from build123d import *

# Parameters (mm, degrees)
F1_W     = 101.6
F1_H     = 101.6
F2_DEPTH = 50.8
F3_W     = 34.3186343089
F3_H     = 34.3186343089
F4_DEPTH = 46.228
F5_W     = 34.3186343089
F5_H     = 34.3186343089
F6_DEPTH = 45.974


# Not quite as in the source:
# - a variable given as a bare number and used for a length is read in inches; the dataset says mm whatever the document's units were


with BuildPart() as f2:
    # F1 (on Front) → F2 (new body, symmetric)
    with BuildSketch(Plane.XZ):
        Rectangle(F1_W, F1_H)
    extrude(amount=F2_DEPTH, both=True)

    # F3 (on face) → F4 (cut)
    with BuildSketch(Plane.XZ.offset(50.8)):
        with Locations((0, 3.3200695179)):
            Rectangle(F3_W, F3_H)
    extrude(amount=-F4_DEPTH, mode=Mode.SUBTRACT)

    # F5 (on face) → F6 (cut)
    with BuildSketch(Plane(origin=(0, 50.8, 0), x_dir=(-1, 0, 0), z_dir=(0, 1, 0))):
        with Locations((0, 3.3200695179)):
            Rectangle(F5_W, F5_H)
    extrude(amount=-F6_DEPTH, mode=Mode.SUBTRACT)


solid = f2.part
Model file for the job. Use its own axes, mm. A direction names the side the tool comes from. Round coordinates to 2 decimals unless told otherwise and drop trailing zeros. Loops run counter-clockwise (first coordinate to the right, second up) from the corner with the lowest first, then second, coordinate; pieces in that order, holes last. Notation, with made-up numbers: (28.5, 11) -> (43.5, 11) arc R32 ccw to (43.5, 45) -> close; hole circle Ø4 at (87.25, -24.5). An arc over 180 degrees is marked (long way). Answer as CSV lines item,"result". Start each with the question number.
1) Slice it at B-B (z = 11). List the corners of the cut face in (x, y).
2) Tool access for faces 1 (the face through (-1, -1, -50.8)), 2 (the face through (17.159, -28, 3)), 3 (the face through (0, 4.826, 4)): list every direction of +Z, -Z, +X, -X, +Y, -Y with a clear straight run to the whole face (end or side of a thin tool).
3) Mould opens along X. For faces 4 (the face through (17.159, 28, 3)), 5 (the face through (50.8, -1, -1)), 6 (the face through (22, 50.8, 1)), 7 (the face through (-50.8, -1, -1)) say: +X half, -X half, draft (parallel to the pull), parting line (faces both ways), or undercut.
4) Pin check, flat tips, straight feed: P1, Ø3, axis at x = 7.5, z = 7, coming from the -Y side; P2, Ø10.5, axis at x = -5.5, z = 6.5, coming from the +Y side. Stop position of each tip, or through.
5) Probe line 1 along Z through (x, y) = (-8, -32); line 2 along X through (y, z) = (-25.5, -13.5); line 3 along Y through (x, z) = (-10.5, -13). List the from-to ranges inside material, lowest first.
6) Slice it at C-C (x = 1). List the corners of the cut face in (y, z), plus the area to 3 significant figures.
7) Slice it at A-A (y = -44). List the corners of the cut face in (x, z), plus the area to 3 significant figures.
Filled in:
1,outline,"(-50.8, -50.8) -> (-17.16, -50.8) -> (-17.16, -4.57) -> (17.16, -4.57) -> (17.16, -50.8) -> (50.8, -50.8) -> (50.8, 50.8) -> (17.16, 50.8) -> (17.16, 4.83) -> (-17.16, 4.83) -> (-17.16, 50.8) -> (-50.8, 50.8) -> close"
2,face 1,"-Z, +X, -X, +Y, -Y"
2,face 2,"-Y"
2,face 3,"+Y"
3,face 4,"undercut"
3,face 5,"+X half"
3,face 6,"draft"
3,face 7,"-X half"
4,P1,"stops at y = -4.57"
4,P2,"stops at y = 4.83"
5,line 1,"z = -50.8 to -13.84, 20.48 to 50.8"
5,line 2,"x = -50.8 to -17.16, 17.16 to 50.8"
5,line 3,"y = -4.57 to 4.83"
6,outline,"(-50.8, -50.8) -> (50.8, -50.8) -> (50.8, -13.84) -> (4.83, -13.84) -> (4.83, 20.48) -> (50.8, 20.48) -> (50.8, 50.8) -> (-50.8, 50.8) -> (-50.8, 20.48) -> (-4.57, 20.48) -> (-4.57, -13.84) -> (-50.8, -13.84) -> close"
6,area,"7,160 mm2"
7,outline,"(-50.8, -50.8) -> (50.8, -50.8) -> (50.8, 50.8) -> (-50.8, 50.8) -> close; hole (-17.16, -13.84) -> (17.16, -13.84) -> (17.16, 20.48) -> (-17.16, 20.48) -> close"
7,area,"9,140 mm2"
